Can you work these out from the model? Positions are in its coordinate system, mm. Coordinates: 2 decimals unless noted, no trailing zeros. Loops run counter-clockwise (first coordinate to the right, second up) from the corner with the lowest first, then second, coordinate; pieces in that order, holes last.
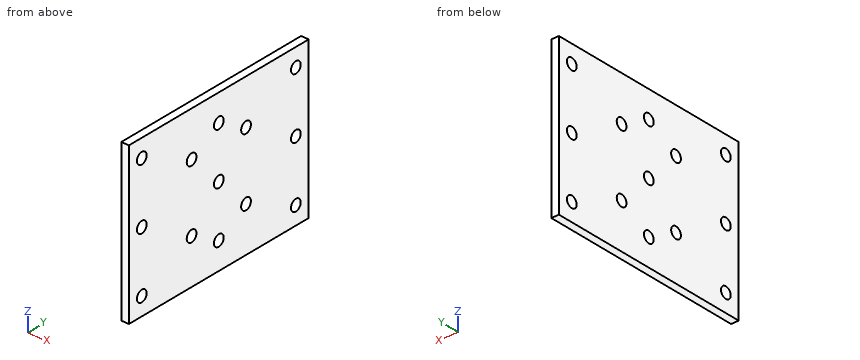
```python
from build123d import *

# Parameters (mm, degrees)
SKETCH11_W                     = 3.4
SKETCH11_H                     = 52
BASE_FLANGE3_DEPTH             = 70
EDGE_FLANGE1_STRIP_W           = 15.1
EDGE_FLANGE1_STRIP_H           = 3.4
EDGE_FLANGE1_STRIP_CUT_DEPTH   = 70
EDGE_FLANGE1_STRIP_2_W         = 15.1
EDGE_FLANGE1_STRIP_2_H         = 3.4
EDGE_FLANGE1_STRIP_CUT_2_DEPTH = 70
EDGE_FLANGE1_DEPTH             = 70
EDGE_FLANGE1_BEND_DEPTH        = 70
CUT_EXTRUDE1_DEPTH             = 89.011135659
CUT_EXTRUDE1_DEPTH_BACK        = 89.011135659
SKETCH25_R                     = 2.5
SKETCH23_R                     = 2.5
CUT_EXTRUDE2_DEPTH             = 77.954272136
UNFOLD1_START                  = -22
UNFOLD1_OUTLINE_W              = 4.15
UNFOLD1_OUTLINE_H              = 70
UNFOLD1_DEPTH                  = 18.6
UNFOLD1_START_2                = -3.4
UNFOLD1_2_OUTLINE_W            = 24.368804756
UNFOLD1_2_OUTLINE_H            = 70
UNFOLD1_2_OUTLINE_R            = 2.5
UNFOLD1_2_DEPTH                = 3.4


with BuildPart() as part:
    # Base-Flange3: sheet metal written as solids
    # Sketch11 → Base-Flange3 (new body)
    with BuildSketch(Plane.XY):
        with Locations((-1.7, 0)):
            Rectangle(SKETCH11_W, SKETCH11_H)
    extrude(amount=BASE_FLANGE3_DEPTH)

    # Edge-Flange1: sheet metal written as solids
    # Edge-Flange1 strip (on a plane across the edge) → Edge-Flange1 strip cut (cut)
    with BuildSketch(Plane(origin=(-3.4, 26, 70), x_dir=(0, -1, 0), z_dir=(0, 0, -1))):
        with Locations((-3.4, -1.7)):
            Rectangle(EDGE_FLANGE1_STRIP_W, EDGE_FLANGE1_STRIP_H)
    extrude(amount=EDGE_FLANGE1_STRIP_CUT_DEPTH, mode=Mode.SUBTRACT)

    # Edge-Flange1 strip 2 (on a plane across the edge) → Edge-Flange1 strip cut 2 (cut)
    with BuildSketch(Plane(origin=(-3.4, -26, 0), x_dir=(0, 1, 0), z_dir=(0, 0, 1))):
        with Locations((-3.4, -1.7)):
            Rectangle(EDGE_FLANGE1_STRIP_2_W, EDGE_FLANGE1_STRIP_2_H)
    extrude(amount=EDGE_FLANGE1_STRIP_CUT_2_DEPTH, mode=Mode.SUBTRACT)

    # Edge-Flange1 section (on a plane across the edge) → Edge-Flange1 (add)
    with BuildSketch(Plane(origin=(-3.4, 26, 70), x_dir=(0, -1, 0), z_dir=(0, 0, -1))):
        with BuildLine():
            Line((0, 0.75), (0, 18.6))
            Line((0, 18.6), (3.4, 18.6))
            Line((3.4, 18.6), (3.4, 0.75))
            ThreePointArc((3.4, 0.75), (3.619669914, 0.219669914), (4.15, 0))
            Line((4.15, 0), (4.15, -3.4))
            ThreePointArc((4.15, -3.4), (1.215506858, -2.184493142), (0, 0.75))
        make_face()
    extrude(amount=EDGE_FLANGE1_DEPTH)

    # Edge-Flange1 section 2 (on a plane across the edge) → Edge-Flange1 bend (add)
    with BuildSketch(Plane(origin=(-3.4, -26, 0), x_dir=(0, 1, 0), z_dir=(0, 0, 1))):
        with BuildLine():
            Line((0, 0.75), (0, 18.6))
            Line((0, 18.6), (3.4, 18.6))
            Line((3.4, 18.6), (3.4, 0.75))
            ThreePointArc((3.4, 0.75), (3.619669914, 0.219669914), (4.15, 0))
            Line((4.15, 0), (4.15, -3.4))
            ThreePointArc((4.15, -3.4), (1.215506858, -2.184493142), (0, 0.75))
        make_face()
    extrude(amount=EDGE_FLANGE1_BEND_DEPTH)

    # Sketch25 → Cut-Extrude1 (cut, two sides: drawn at the far end of the back side and taken through both)
    with BuildSketch(Plane.XZ.offset(-22.6).offset(-CUT_EXTRUDE1_DEPTH_BACK)):
        with Locations((-15.4, 35)):
            Circle(SKETCH25_R)
        with Locations((-15.4, 8)):
            Circle(SKETCH25_R)
        with Locations(Location((-15.4, 62, 0), (0, 0, 180))):
            Circle(SKETCH25_R)
    extrude(amount=CUT_EXTRUDE1_DEPTH + CUT_EXTRUDE1_DEPTH_BACK, mode=Mode.SUBTRACT)

    # Sketch23 → Cut-Extrude2 (cut, through all)
    with BuildSketch(Plane.ZY.offset(3.4)):
        with Locations(Location((20, -14, 0), (0, 0, 270))):
            Circle(SKETCH23_R)
        with Locations(Location((50, -14, 0), (0, 0, 270))):
            Circle(SKETCH23_R)
        with Locations(Location((20, 14, 0), (0, 0, 90))):
            Circle(SKETCH23_R)
        with Locations(Location((50, 14, 0), (0, 0, 270))):
            Circle(SKETCH23_R)
        with Locations(Location((35, 0, 0), (0, 0, 270))):
            Circle(SKETCH23_R)
        with Locations(Location((58, 0, 0), (0, 0, 270))):
            Circle(SKETCH23_R)
        with Locations(Location((12, 0, 0), (0, 0, 90))):
            Circle(SKETCH23_R)
    extrude(amount=-CUT_EXTRUDE2_DEPTH, mode=Mode.SUBTRACT)

    # Unfold1: read off the stored shape, not the designer's step
    # Unfold1 outline → Unfold1 (cut)
    with BuildSketch(Plane.YZ.offset(UNFOLD1_START)):
        with Locations((-23.925, 35)):
            Rectangle(UNFOLD1_OUTLINE_W, UNFOLD1_OUTLINE_H)
        with Locations((23.925, 35)):
            Rectangle(UNFOLD1_OUTLINE_W, UNFOLD1_OUTLINE_H)
    extrude(amount=UNFOLD1_DEPTH, mode=Mode.SUBTRACT)

    # Unfold1 2 outline → Unfold1 2 (add)
    # profile 1 of 2: a face of its own
    with BuildSketch(Plane.YZ.offset(UNFOLD1_START_2)):
        with Locations((-34.034402378, 35)):
            Rectangle(UNFOLD1_2_OUTLINE_W, UNFOLD1_2_OUTLINE_H)
        with Locations((-39.618804756, 8)):
            Circle(UNFOLD1_2_OUTLINE_R, mode=Mode.SUBTRACT)
        with Locations((-39.618804756, 35)):
            Circle(UNFOLD1_2_OUTLINE_R, mode=Mode.SUBTRACT)
        with Locations((-39.618804756, 62)):
            Circle(UNFOLD1_2_OUTLINE_R, mode=Mode.SUBTRACT)
    # profile 2 of 2: a face of its own
    with BuildSketch(Plane.YZ.offset(UNFOLD1_START_2)):
        with Locations((34.034402378, 35)):
            Rectangle(UNFOLD1_2_OUTLINE_W, UNFOLD1_2_OUTLINE_H)
        with Locations((39.618804756, 8)):
            Circle(UNFOLD1_2_OUTLINE_R, mode=Mode.SUBTRACT)
        with Locations((39.618804756, 35)):
            Circle(UNFOLD1_2_OUTLINE_R, mode=Mode.SUBTRACT)
        with Locations((39.618804756, 62)):
            Circle(UNFOLD1_2_OUTLINE_R, mode=Mode.SUBTRACT)
    extrude(amount=UNFOLD1_2_DEPTH)


solid = part.part
```
(1) I want a section at D-D on z = 35. Write out the boundary of the cut face in (x, y), then the cut area to 3 significant figures.
Check values:
outline: (-3.4, -46.22) - (0, -46.22) - (0, -42.12) - (-3.4, -42.12) - close; (-3.4, -37.12) - (0, -37.12) - (0, -2.5) - (-3.4, -2.5) - close; (-3.4, 2.5) - (0, 2.5) - (0, 37.12) - (-3.4, 37.12) - close; (-3.4, 42.12) - (0, 42.12) - (0, 46.22) - (-3.4, 46.22) - close
area: 263 mm2
(2) I want a section at A-A on z = 50. Write out the boundary of the cut face in (x, y), then the cut area to 3 significant figures.
Check values:
outline: (-3.4, -46.22) - (0, -46.22) - (0, -16.5) - (-3.4, -16.5) - close; (-3.4, -11.5) - (0, -11.5) - (0, 11.5) - (-3.4, 11.5) - close; (-3.4, 16.5) - (0, 16.5) - (0, 46.22) - (-3.4, 46.22) - close
area: 280 mm2
(3) If I drill on probe 1 along Z at (x, y) = (-2.05, -14); probe 2 along Z at (x, y) = (-1.1, 0); probe 3 along Y at (x, z) = (-1.3, 51), over which ranges is the centre line in solid material (lowest first)?
Check values:
probe 1: z = 0 to 17.5, 22.5 to 47.5, 52.5 to 70
probe 2: z = 0 to 9.5, 14.5 to 32.5, 37.5 to 55.5, 60.5 to 70
probe 3: y = -46.22 to -16.29, -11.71 to 11.71, 16.29 to 46.22
(4) I want a section at B-B on y = 0. Write out the boundary of the cut face in (x, z), then the cut area to 3 significant figures.
Check values:
outline: (-3.4, 0) - (0, 0) - (0, 9.5) - (-3.4, 9.5) - close; (-3.4, 14.5) - (0, 14.5) - (0, 32.5) - (-3.4, 32.5) - close; (-3.4, 37.5) - (0, 37.5) - (0, 55.5) - (-3.4, 55.5) - close; (-3.4, 60.5) - (0, 60.5) - (0, 70) - (-3.4, 70) - close
area: 187 mm2
(5) I'm going to push a flat-ended pin straight in: pin 1 (4.5 mm diameter, centred on y = 39.62, z = 35, fed in from +X). Where does the tip first touch, or does it pass through?
Check values:
pin 1: passes through
(6) I want a section at C-C on x = -1.85. State how many separate pieces and enclosed holes the cut face has, then the cut area to 3 significant figures.
Check values:
separate pieces: 1
enclosed holes: 13
area: 6,220 mm2
